```python
from build123d import *

# Parameters (mm, degrees)
SKETCH1_W           = 50.8
SKETCH1_H           = 50.8
BOSS_EXTRUDE1_DEPTH = 10.16
SKETCH2_R           = 2.286
CUT_EXTRUDE1_DEPTH  = 38.33022368
SKETCH3_R           = 3.429
CUT_EXTRUDE2_DEPTH  = 6.35
SKETCH4_R           = 3.429
CUT_EXTRUDE3_DEPTH  = 38.33022368
SKETCH5_R           = 1.905
CUT_EXTRUDE5_DEPTH  = 38.33022368


with BuildPart() as part:
    # Sketch1 → Boss-Extrude1 (new body)
    with BuildSketch(Plane(origin=(0, 0, 0), x_dir=(1, 0, 0), z_dir=(0, 1, 0))):
        Rectangle(SKETCH1_W, SKETCH1_H)
    extrude(amount=BOSS_EXTRUDE1_DEPTH)

    # Sketch2 → Cut-Extrude1 (cut, through all)
    with BuildSketch(Plane(origin=(0, 10.16, 0), x_dir=(1, 0, 0), z_dir=(0, 1, 0))):
        with Locations(Location((-19.05, 12.7, 0), (0, 0, 270))):
            Circle(SKETCH2_R)
        with Locations(Location((19.05, 12.7, 0), (0, 0, 270))):
            Circle(SKETCH2_R)
        with Locations(Location((0, -12.7, 0), (0, 0, 270))):
            Circle(SKETCH2_R)
    extrude(amount=-CUT_EXTRUDE1_DEPTH, mode=Mode.SUBTRACT)

    # Sketch3 → Cut-Extrude2 (cut)
    # profile 1 of 3: a face of its own
    with BuildSketch(Plane.XZ):
        with BuildLine():
            Line((-6.35, 16.256), (-6.35, 5.08))
            ThreePointArc((-6.35, 5.08), (-13.97, -2.54), (-21.59, 5.08))
            Line((-21.59, 5.08), (-21.59, 16.256))
            ThreePointArc((-21.59, 16.256), (-13.97, 23.876), (-6.35, 16.256))
        make_face()
        with Locations(Location((-13.97, 10.668, 0), (0, 0, 270))):
            Circle(SKETCH3_R, mode=Mode.SUBTRACT)
    # profile 2 of 3: a face of its own
    with BuildSketch(Plane.XZ):
        with BuildLine():
            Line((21.59, 16.256), (21.59, 5.08))
            ThreePointArc((21.59, 5.08), (13.97, -2.54), (6.35, 5.08))
            Line((6.35, 5.08), (6.35, 16.256))
            ThreePointArc((6.35, 16.256), (13.97, 23.876), (21.59, 16.256))
        make_face()
        with Locations(Location((13.97, 10.668, 0), (0, 0, 270))):
            Circle(SKETCH3_R, mode=Mode.SUBTRACT)
    # profile 3 of 3: a face of its own
    with BuildSketch(Plane.XZ):
        with BuildLine():
            Line((-5.588, -7.112), (5.588, -7.112))
            ThreePointArc((5.588, -7.112), (13.208, -14.732), (5.588, -22.352))
            Line((5.588, -22.352), (-5.588, -22.352))
            ThreePointArc((-5.588, -22.352), (-13.208, -14.732), (-5.588, -7.112))
        make_face()
        with Locations(Location((0, -14.732, 0), (0, 0, 270))):
            Circle(SKETCH3_R, mode=Mode.SUBTRACT)
    extrude(amount=-CUT_EXTRUDE2_DEPTH, mode=Mode.SUBTRACT)

    # Sketch4 → Cut-Extrude3 (cut, through all)
    with BuildSketch(Plane(origin=(0, 0, 0), x_dir=(-1, 0, 0), z_dir=(0, -1, 0))):
        with Locations(Location((13.97, -10.668, 0), (0, 0, 90))):
            Circle(SKETCH4_R)
        with Locations(Location((-13.97, -10.668, 0), (0, 0, 90))):
            Circle(SKETCH4_R)
        with Locations(Location((0, 14.732, 0), (0, 0, 90))):
            Circle(SKETCH4_R)
    extrude(amount=-CUT_EXTRUDE3_DEPTH, mode=Mode.SUBTRACT)

    # Sketch5 → Cut-Extrude5 (cut, through all)
    with BuildSketch(Plane(origin=(0, 10.16, 0), x_dir=(1, 0, 0), z_dir=(0, 1, 0))):
        with Locations(Location((0, 0, 0), (0, 0, 270))):
            Circle(SKETCH5_R)
    extrude(amount=-CUT_EXTRUDE5_DEPTH, mode=Mode.SUBTRACT)


solid = part.part
```
The listing builds one solid part. Answer for the finished solid, in the listing's coordinates (mm). A direction names the side the tool comes from. Round coordinates to 2 decimals unless told otherwise and drop trailing zeros. Order: outer loops, then holes, each group sorted by start corner. A loop starts at its lowest first (then second) coordinate and runs counter-clockwise, first axis right, second up. Notation, with made-up numbers: (41.25, 42.5) - (54.25, 42.5) arc R28 ccw to (54.25, 63.5) - close; hole circle Ø9 at (12, 82.25). An arc over 180 degrees is marked (long way). Put each result on its own line as item: value. Start each with the question number.
(1) Determine the mould class of faces 1 (the flat face through (5, 10.16, 0)), 2 (the flat face through (-25.4, 5, 0)), 3 (the flat face through (0, 6.35, -11)) for opening direction X: released by +X, released by -X, zero draft, split by the parting line, or undercut.
(2) Find section B-B (y = 8.5). Give the vertices of the cut face in (x, z) (3 decimals).
(3) Find section A-A (x = 13.97). Give the vertices of the cut face in (y, z), plus the area to 3 significant figures.
(4) For faces 4 (the cylindrical face through (1.89, 5.15, -0.25)), 5 (the cylindrical face through (13.206, 3.131, -14.564)), determine the directions among +Z, -Z, +X, -X, +Y, -Y from which every point of the face is accessible in a straight line to the end or side of a thin tool.
(5) Find section C-C (z = 0). Give the vertices of the cut face in (x, y) (3 decimals).
(6) Find section D-D (x = 1). Give the vertices of the cut face in (y, z), plus the area to 3 significant figures.
(7) Given P1, Ø12, axis at x = 15.5, z = 7.5, coming from the -Y side; P2, Ø4, axis at x = 13.97, z = 10.668, coming from the +Y side, each flat-ended and moving along its own axis, determine where each tip first touches the part or whether it passes through.
(8) Straight lines are drawn through the part: probe 1 along Z at (x, y) = (5.5, 1.5); probe 2 along Z at (x, y) = (1.5, 1.25); probe 3 along X at (y, z) = (4.25, -12.7). For each, find the intervals that lie inside material, in ascending order. Write a range as from..to.
Reply:
1. face 1: zero draft
1. face 2: released by -X
1. face 3: undercut
2. outline: (-25.4, -25.4) - (25.4, -25.4) - (25.4, 25.4) - (-25.4, 25.4) - close; hole circle Ø4.572 at (-19.05, -12.7); hole circle Ø6.858 at (-13.97, 10.668); hole circle Ø6.858 at (0, -14.732); hole circle Ø4.572 at (0, 12.7); hole circle Ø3.81 at (0, 0); hole circle Ø6.858 at (13.97, 10.668); hole circle Ø4.572 at (19.05, -12.7)
3. outline: (0, -25.4) - (10.16, -25.4) - (10.16, 7.24) - (6.35, 7.24) - (6.35, -2.54) - (0, -2.54) - close; (0, 23.88) - (6.35, 23.88) - (6.35, 14.1) - (10.16, 14.1) - (10.16, 25.4) - (0, 25.4) - close
3. area: 322 mm^2
4. face 4: +Y, -Y
4. face 5: -Y
5. outline: (-25.4, 0) - (-19.65, 0) - (-19.65, 6.35) - (-8.29, 6.35) - (-8.29, 0) - (-1.905, 0) - (-1.905, 10.16) - (-25.4, 10.16) - close; (1.905, 0) - (8.29, 0) - (8.29, 6.35) - (19.65, 6.35) - (19.65, 0) - (25.4, 0) - (25.4, 10.16) - (1.905, 10.16) - close
6. outline: (0, -25.4) - (10.16, -25.4) - (10.16, -18.01) - (6.35, -18.01) - (6.35, -22.35) - (0, -22.35) - close; (0, -7.11) - (6.35, -7.11) - (6.35, -11.45) - (10.16, -11.45) - (10.16, -1.62) - (0, -1.62) - close; (0, 1.62) - (10.16, 1.62) - (10.16, 10.64) - (0, 10.64) - close; (0, 14.76) - (10.16, 14.76) - (10.16, 25.4) - (0, 25.4) - close
6. area: 320 mm^2
7. P1: y = 6.35
7. P2: through
8. probe 1: -25.4..-22.35, -7.11..25.4
8. probe 2: -25.4..-22.35, -7.11..-1.17, 1.17..10.97, 14.43..25.4
8. probe 3: -25.4..-21.34, -16.76..-12.93, 12.93..16.76, 21.34..25.4
